Here's how the part is built. I have some questions about the finished solid (model axes, mm). Face numbers are marked on the shaded views. A direction names the side the tool comes from. Round coordinates to 2 decimals unless told otherwise and drop trailing zeros. Loops run counter-clockwise (first coordinate to the right, second up) from the corner with the lowest first, then second, coordinate; pieces in that order, holes last. Notation, with made-up numbers: M -19.75,-34 L -2.75,-34 A19 ccw -2.75,2 Z; hole C 85.25,25.5 d4. An arc over 180 degrees is marked long. Write each question's results on one line, items separated by ' | '. Start each with the question number.
```python
from build123d import *

# Parameters (mm, degrees)
SKETCH1_W           = 64
SKETCH1_H           = 45
BOSS_EXTRUDE1_DEPTH = 2.5
SKETCH3_W           = 17
SKETCH3_H           = 20.5
BOSS_EXTRUDE2_DEPTH = 2.5
BOSS_EXTRUDE4_DEPTH = 2.5
SKETCH6_R           = 5
BOSS_EXTRUDE5_DEPTH = 1
BOSS_EXTRUDE6_DEPTH = 5
SKETCH8_R           = 1.5
CUT_EXTRUDE1_DEPTH  = 2.5
SKETCH9_R           = 4.75
BOSS_EXTRUDE7_DEPTH = 3.5
SKETCH10_R          = 2.6
BOSS_EXTRUDE8_DEPTH = 4.5
SKETCH11_R          = 1.5
CUT_EXTRUDE2_DEPTH  = 2
SKETCH12_R          = 1.5
CUT_EXTRUDE3_DEPTH  = 2


with BuildPart() as part:
    # Sketch1 → Boss-Extrude1 (new body)
    with BuildSketch(Plane.XY):
        with Locations((0, -2.648063781)):
            Rectangle(SKETCH1_W, SKETCH1_H)
    extrude(amount=BOSS_EXTRUDE1_DEPTH)

    # Sketch3 → Boss-Extrude2 (add)
    with BuildSketch(Plane.XZ.offset(25.148063781)):
        with Locations((-23.5, -7.75)):
            Rectangle(SKETCH3_W, SKETCH3_H)
        with Locations((23.5, -7.75)):
            Rectangle(SKETCH3_W, SKETCH3_H)
    extrude(amount=BOSS_EXTRUDE2_DEPTH)

    # Sketch5 → Boss-Extrude4 (add)
    with BuildSketch(Plane.XY.offset(2.5)):
        with BuildLine():
            Line((-12, -25.148063781), (-12, -31.648063781))
            ThreePointArc((-12, -31.648063781), (0, -43.648063781), (12, -31.648063781))
            Line((12, -31.648063781), (12, -25.148063781))
            Line((12, -25.148063781), (-12, -25.148063781))
        make_face()
    extrude(amount=-BOSS_EXTRUDE4_DEPTH)

    # Sketch6 → Boss-Extrude5 (add)
    with BuildSketch(Plane.XY.offset(2.5)):
        with Locations((0, -31.648063781)):
            Circle(SKETCH6_R)
    extrude(amount=BOSS_EXTRUDE5_DEPTH)

    # Sketch7 → Boss-Extrude6 (add)
    with BuildSketch(Plane.XY.offset(3.5)):
        Polygon((0.007672283, -27.164333449), (-3.933372225, -29.439696556), (-3.933372225, -33.990422772), (0.007672283, -36.26578588), (3.948716792, -33.990422772), (3.948716792, -29.439696556), align=None)
    extrude(amount=BOSS_EXTRUDE6_DEPTH)

    # Sketch8 → Cut-Extrude1 (cut)
    with BuildSketch(Plane.XY.offset(2.5)):
        with Locations((-20, -13.148063781)):
            Circle(SKETCH8_R)
        with Locations((-1, 5.851936219)):
            Circle(SKETCH8_R)
    extrude(amount=-CUT_EXTRUDE1_DEPTH, mode=Mode.SUBTRACT)

    # Sketch9 → Boss-Extrude7 (add)
    with BuildSketch(Plane.XY.offset(2.5)):
        with Locations((-20, 7.851936219)):
            Circle(SKETCH9_R)
        with Locations((20, 7.851936219)):
            Circle(SKETCH9_R)
    extrude(amount=BOSS_EXTRUDE7_DEPTH)

    # Sketch10 → Boss-Extrude8 (add)
    with BuildSketch(Plane.XY.offset(2.5)):
        with Locations((10, -4.148063781)):
            Circle(SKETCH10_R)
        with Locations((23.5, -4.148063781)):
            Circle(SKETCH10_R)
    extrude(amount=BOSS_EXTRUDE8_DEPTH)

    # Sketch11 → Cut-Extrude2 (cut)
    with BuildSketch(Plane.XY.offset(7)):
        with Locations((10, -4.148063781)):
            Circle(SKETCH11_R)
    extrude(amount=-CUT_EXTRUDE2_DEPTH, mode=Mode.SUBTRACT)

    # Sketch12 → Cut-Extrude3 (cut)
    with BuildSketch(Plane.XY.offset(7)):
        with Locations((23.5, -4.148063781)):
            Circle(SKETCH12_R)
    extrude(amount=-CUT_EXTRUDE3_DEPTH, mode=Mode.SUBTRACT)


solid = part.part
```
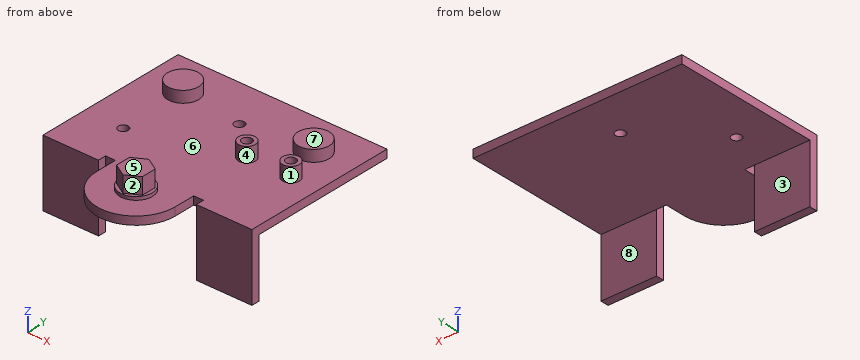
Item 1: If we section it at B-B on x = -20: Please give me the cut outline in (y, z).
Item 2: If we section it at D-D on y = -18.5: Please give me the cut outline in (x, z).
Item 3: I need wall thicknesses on L1, parallel to X at y = -13, z = 1.5; L2, parallel to Z at x = 10, y = -16; L3, parallel to Y at x = -20, z = 1.7. Which ranges of each line are inside material? Lowest first, please.
Item 4: I'm going to push flat-ended pins straight in: pin 1 (5 mm diameter, centred on y = -31, z = 5.5, fed in from -X); pin 2 (19 mm diameter, centred on x = 5, y = -9.5, fed in from +Z); pin 3 (5 mm diameter, centred on x = -27, z = -7, fed in from +Y). Where does each tip first touch, or does it pass through?
Item 5: If we section it at A-A on z = -5.25: Please give me the cut outline in (x, y), and give its area (3 significant figures).
Item 6: If we mould it in two halves opening along X, with no side actions, what happens to the marked faces 1, 2, 3 and 4? For each: released by +X, released by -X, zero draft, split by the parting line, or undercut.
Item 7: Which directions (+Z, -Z, +X, -X, +Y, -Y) give clear straight access to the entire face, cutting with the end or side of a thin tool? Please do the marked faces 5, 6, 7 and 8.
Item 8: If we section it at C-C on x = 20: Please give me the cut outline in (y, z), and give its area (3 significant figures).
Numbers:
1) outline: M -27.65,-18 L -25.15,-18 L -25.15,0 L -14.65,0 L -14.65,2.5 L -27.65,2.5 Z; M -11.65,0 L 19.85,0 L 19.85,2.5 L 12.6,2.5 L 12.6,6 L 3.1,6 L 3.1,2.5 L -11.65,2.5 Z
2) outline: M -32,0 L 32,0 L 32,2.5 L -32,2.5 Z
3) L1: -32 to -21.49, -18.51 to 32 | L2: 0 to 2.5 | L3: -27.65 to -14.65, -11.65 to 19.85
4) pin 1: x = -5 | pin 2: z = 7 | pin 3: y = -25.15
5) outline: M -32,-27.65 L -15,-27.65 L -15,-25.15 L -32,-25.15 Z; M 15,-27.65 L 32,-27.65 L 32,-25.15 L 15,-25.15 Z | area: 85.0 mm²
6) face 1: undercut | face 2: released by +X | face 3: zero draft | face 4: undercut
7) face 5: +Z, +X, -X, +Y, -Y | face 6: +Z | face 7: +Z, +X, -X, +Y | face 8: -Z, +X, -X, +Y
8) outline: M -27.65,-18 L -25.15,-18 L -25.15,0 L 19.85,0 L 19.85,2.5 L 12.6,2.5 L 12.6,6 L 3.1,6 L 3.1,2.5 L -27.65,2.5 Z | area: 197 mm²
